Part print with two shaded views. Sizes in mm from the minimum x, y, z corner. A direction names the side the tool comes from. Coordinates: 2 decimals unless noted, no trailing zeros. Write each question's results on one line, items separated by ' | '. Start each with the question number.
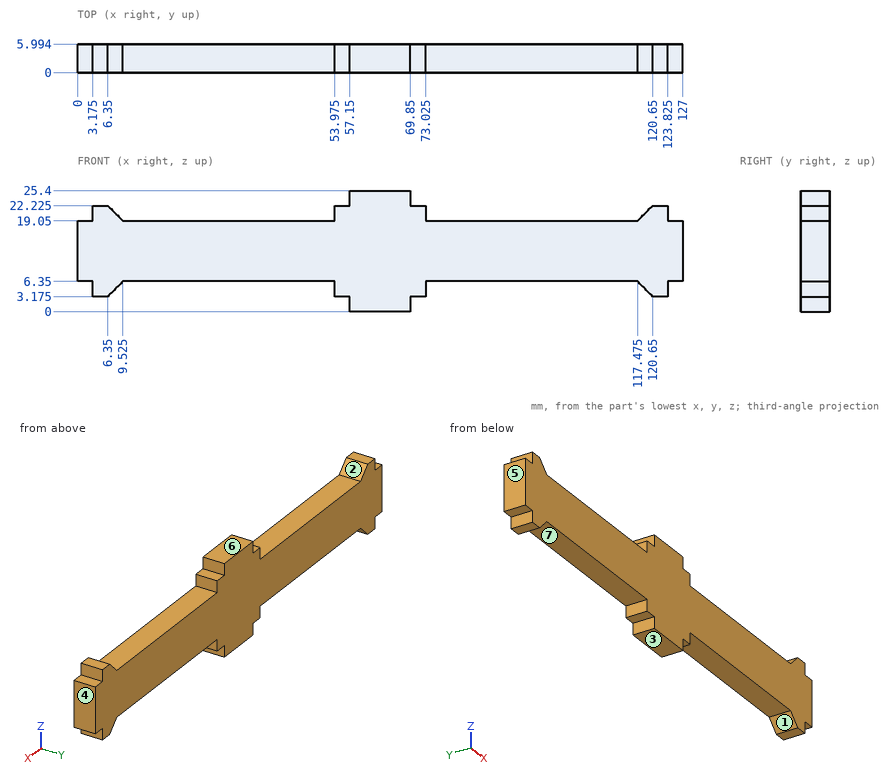
Q1. Mould opens along X. For the marked faces 4, 5, 6 and 7 say: +X half, -X half, draft (parallel to the pull), parting line (faces both ways), or undercut.
Q2. Pin check, flat tips, straight feed: pin 1 (1 mm diameter, centred on x = 5, y = 4, fed in from -Z) (3 decimals); pin 2 (1 mm diameter, centred on x = 55.5, y = 4.5, fed in from +Z) (3 decimals); pin 3 (1 mm diameter, centred on x = 125, y = 3.5, fed in from +Z). Stop position of each tip, or through.
Q3. Drill centre lines: L1, parallel to X at y = 2.5, z = 20.75 (1 decimal); L2, parallel to X at y = 0.4, z = 4.5 (1 decimal); L3, parallel to Z at x = 42, y = 5.4. Where is each one in solid material? Low to high. Write a range as from..to.
Q4. Which spindle directions (+Z, -Z, +X, -X, +Y, -Y) get a long thin tool onto all of the face, cutting with end or side? Do the marked faces 1, 2 and 3. Say none if no direction does.
Check result:
1) face 4: +X half | face 5: -X half | face 6: draft | face 7: undercut
2) pin 1: z = 3.175 | pin 2: z = 22.225 | pin 3: z = 19.05
3) L1: 3.2..7.8, 54..73, 119.2..123.8 | L2: 3.2..7.7, 54..73, 119.3..123.8 | L3: 6.35..19.05
4) face 1: -Z, +Y, -Y | face 2: +Z, +Y, -Y | face 3: -Z, +X, -X, +Y, -Y
